Work out the finished part from the listing and answer in its coordinate system (mm). A direction names the side the tool comes from. Round coordinates to 2 decimals unless told otherwise and drop trailing zeros. Loops run counter-clockwise (first coordinate to the right, second up) from the corner with the lowest first, then second, coordinate; pieces in that order, holes last. Notation, with made-up numbers: (-31.5, -0.75) - (17.5, -0.75) arc R19 ccw to (17.5, 5.25) - close; hole circle Ø6 at (-26, 8.5). An arc over 180 degrees is marked (long way). Return JSON: item names as keys, results as strings.
from build123d import *

# Parameters (mm, degrees)
F0_W          = 127
F0_H          = 76.2
F1_DEPTH      = 25.4
F1_DEPTH_BACK = 25.4
F2_R          = 12.7
F3_DEPTH      = 44.45
F4_R          = 12.7
F5_DEPTH      = 44.45


# Not quite as in the source:
# - a feature names something its author has since deleted; it is built from what else it names


with BuildPart() as f1:
    # F0 (on Front) → F1 (new body, two sides)
    with BuildSketch(Plane.XZ) as f1_sk:
        with Locations((1.2215264142, -26.8060624134)):
            Rectangle(F0_W, F0_H)
    extrude(amount=F1_DEPTH)
    extrude(f1_sk.sketch, amount=-F1_DEPTH_BACK)

    # F2 (on face) → F3 (cut)
    with BuildSketch(Plane.XZ.offset(25.4)):
        with Locations((1.2215264142, -26.8060624134)):
            Circle(F2_R)
    extrude(amount=-F3_DEPTH, mode=Mode.SUBTRACT)

    # F4 (on face) → F5 (cut)
    with BuildSketch(Plane.YZ.offset(64.7215264142)):
        with Locations((0, -26.8060624134)):
            Circle(F4_R)
    extrude(amount=-F5_DEPTH, mode=Mode.SUBTRACT)


solid = f1.part
1) Find the intervals of material crossed by L1, parallel to Z at x = 51, y = 0; L2, parallel to Z at x = -5, y = -1; L3, parallel to Y at x = 25.5, z = -34.5, in increasing order.
Verdict:
{"L1": "z = -64.91 to -39.51, -14.11 to 11.29", "L2": "z = -64.91 to -37.88, -15.73 to 11.29", "L3": "y = -25.4 to -10.1, 10.1 to 25.4"}
2) A tool of negligible diameter and unlimited length cuts with its end or side. For faces 4 (the cylindrical face through (-1.532, -3.486, -39.204)), 5 (the flat face through (20.272, 0, -27)), 6 (the flat face through (0, 25.4, -26)), from which of +Z, -Z, +X, -X, +Y, -Y can it reach the whole face along a straight path? Write none if from no direction.
Verdict:
{"face 4": "-Y", "face 5": "+X", "face 6": "+Z, -Z, +X, -X, +Y"}
3) Section C-C (y = -7.5) is taken. Give the vertices of the cut face in (x, z).
Verdict:
{"outline": "(-62.28, -64.91) - (64.72, -64.91) - (64.72, -37.05) - (20.27, -37.05) - (20.27, -16.56) - (64.72, -16.56) - (64.72, 11.29) - (-62.28, 11.29) - close; hole circle Ø25.4 at (1.22, -26.81)"}
4) A flat-ended cylindrical pin translates along its axis: pin 1 (20.5 mm diameter, centred on y = 0, z = -26.81, fed in from +X). Find the tip coordinate at first contact, or state that the pin passes through.
Verdict:
{"pin 1": "stops at x = 20.27"}
5) Determine the mould class of faces 1 (the flat face through (-62.278, 0, -27)), 2 (the flat face through (1, 19.05, -27)), 3 (the flat face through (0, 0, -64.906)) for opening direction Z: pulls with the +Z half, pulls with the -Z half, needs draft (parallel to the pull), parting line crosses it, or undercut.
Verdict:
{"face 1": "needs draft", "face 2": "undercut", "face 3": "pulls with the -Z half"}
6) Section D-D (y = 17) is taken. Give the vertices of the cut face in (x, z), and give its area (3 significant figures).
Verdict:
{"outline": "(-62.28, -64.91) - (64.72, -64.91) - (64.72, 11.29) - (-62.28, 11.29) - close; hole circle Ø25.4 at (1.22, -26.81)", "area": "9,170 mm2"}
7) Section B-B (x = -1) is taken. Give the vertices of the cut face in (y, z), and give its area (3 significant figures).
Verdict:
{"outline": "(-25.4, -64.91) - (25.4, -64.91) - (25.4, 11.29) - (-25.4, 11.29) - (-25.4, -14.3) - (19.05, -14.3) - (19.05, -39.31) - (-25.4, -39.31) - close", "area": "2,760 mm2"}
8) Section A-A (y = -1) is taken. Give the vertices of the cut face in (x, z), and give its area (3 significant figures).
Verdict:
{"outline": "(-62.28, -64.91) - (64.72, -64.91) - (64.72, -39.47) - (20.27, -39.47) - (20.27, -14.15) - (64.72, -14.15) - (64.72, 11.29) - (-62.28, 11.29) - close; hole circle Ø25.4 at (1.22, -26.81)", "area": "8,050 mm2"}
